Work out the finished part from the listing and answer in its coordinate system (mm). A direction names the side the tool comes from. Round coordinates to 2 decimals unless told otherwise and drop trailing zeros. Loops run counter-clockwise (first coordinate to the right, second up) from the corner with the lowest first, then second, coordinate; pieces in that order, holes last. Notation, with made-up numbers: (55, 6) -> (62, 6) arc R34 cw to (62, 39) -> close; hole circle Ø3 at (7.25, -35.75). An arc over 180 degrees is marked (long way). Use one line per item in the form item = value.
```python
from build123d import *

# Parameters (mm, degrees)
SKETCH_W            = 105
SKETCH_H            = 30
PAD_DEPTH           = 100
FILLET_R            = 4
SKETCH001_W         = 4
SKETCH001_H         = 12
POCKET_DEPTH        = 5
LINEARPATTERN_COUNT = 7
LINEARPATTERN_PITCH = 13.333333
SKETCH002_R         = 4
SKETCH002_W         = 27
SKETCH002_H         = 11
POCKET001_DEPTH     = 5


with BuildPart() as part:
    # Sketch → Pad (new body)
    with BuildSketch(Plane.XY):
        Rectangle(SKETCH_W, SKETCH_H)
    extrude(amount=PAD_DEPTH)

    # Fillet
    fillet_edges = [part.edges().sort_by_distance(p)[0] for p in [
        (52.5, 15, 50),
        (52.5, -15, 50),
        (-52.5, 15, 50),
        (-52.5, -15, 50),
    ]]
    fillet(fillet_edges, radius=FILLET_R)

    # Sketch001 (on Face5 of Fillet) → Pocket (cut)
    with BuildSketch(Plane.XY.offset(100)):
        with Locations((-40.5, 0)):
            Rectangle(SKETCH001_W, SKETCH001_H)
    pocket = extrude(amount=-POCKET_DEPTH, mode=Mode.SUBTRACT)

    # LinearPattern: Pocket ×7
    with Locations(*[(i * LINEARPATTERN_PITCH, 0, 0) for i in range(1, LINEARPATTERN_COUNT)]):
        add(pocket, mode=Mode.SUBTRACT)

    # Sketch002 (on Face2 of LinearPattern) → Pocket001 (cut)
    with BuildSketch(Plane(origin=(0, 0, 0), x_dir=(1, 0, 0), z_dir=(0, 0, -1))):
        with Locations((30.333276, 0)):
            Circle(SKETCH002_R)
        with Locations((3.195694, 0)):
            Rectangle(SKETCH002_W, SKETCH002_H)
    extrude(amount=-POCKET001_DEPTH, mode=Mode.SUBTRACT)


solid = part.part
```
(1) For a pull along Y with two mould halves and no side action, classify faces 1 (the flat face through (24.167, 0, 98)), 2 (the flat face through (-1, 7, 0)) as +Y half, -Y half, draft (parallel to the pull), parting line (faces both ways), or undercut.
Completed:
face_1 = undercut
face_2 = draft
(2) For faces 3 (the flat face through (3, 0, 5)), 4 (the flat face through (-1, 7, 100)), 5 (the flat face through (-1, 6, 98)), determine the directions among +Z, -Z, +X, -X, +Y, -Y from which every point of the face is accessible in a straight line to the end or side of a thin tool.
Completed:
face_3 = -Z
face_4 = +Z, +X, -X, +Y, -Y
face_5 = +Z
(3) Consider L1, parallel to X at y = 0, z = 3.5; L2, parallel to Z at x = 12.5, y = 0.5; L3, parallel to Z at x = -5, y = 5. Determine where each line is inside the solid, lowest interval first.
Completed:
L1 = -52.5 to -10.3, 16.7 to 26.33, 34.33 to 52.5
L2 = 5 to 95
L3 = 5 to 100
(4) Given P1, Ø2, axis at x = -14.5, y = -2.5, coming from the +Z side, flat-ended and moving along its own axis, determine where the tip first touches the part or whether it passes through.
Completed:
P1 = 95
(5) Find section A-A, the plane x = -7.5. Write down the section's boundary in (y, z), then the cut area to 4 significant figures.
Completed:
outline = (-15, 0) -> (-5.5, 0) -> (-5.5, 5) -> (5.5, 5) -> (5.5, 0) -> (15, 0) -> (15, 100) -> (-15, 100) -> close
area = 2,945 mm2
